```python
from build123d import *

# Parameters (mm, degrees)
F0_R     = 18.527319
F1_DEPTH = 25.4
F3_DEPTH = 77.216
F5_W     = 28.118574
F5_H     = 19.64978
F6_DEPTH = 25.4


with BuildPart() as f1:
    # F0 (on Top) → F1 (new body)
    with BuildSketch(Plane.XY):
        Circle(F0_R)
    extrude(amount=F1_DEPTH)

    # F2 (on face) → F3 (join)
    with BuildSketch(Plane.XY.offset(25.4)):
        Polygon((6.063722, 17.506937), (-9.906806, 15.656205), (-18.417307, 2.016032), (-13.0592, -13.142255), (2.132751, -18.404156), (15.718697, -9.807352), (17.468143, 6.174588), align=None)
    extrude(amount=F3_DEPTH)

    # F5 (on face) → F6 (join)
    with BuildSketch(Plane.XY.offset(102.616)):
        Rectangle(F5_W, F5_H)
    extrude(amount=F6_DEPTH)


solid = f1.part
```
Geometry check sheet. Reference: the model listing, model coordinates, mm. A direction names the side the tool comes from. Coordinates: 2 decimals unless noted, no trailing zeros. Order: outer loops, then holes, each group sorted by start corner. A loop starts at its lowest first (then second) coordinate and runs counter-clockwise, first axis right, second up.
Q1. Thickness scan on probe 1 along Z at (x, y) = (-1, -17); probe 2 along Y at (x, z) = (6, 119.5); probe 3 along X at (y, z) = (-4, 115). Record the ranges inside material, lowest first.
Reply:
probe 1: z = 0 to 102.62
probe 2: y = -9.82 to 9.82
probe 3: x = -14.06 to 14.06
Q2. Tool access check on faces 1 (the face through (-2, 17, 25.4)), 2 (the face through (0, 13, 102.616)), 3 (the face through (-16, -6, 25.4)), 4 (the face through (14.059, 0, 115)), 5 (the face through (8.831, -14.166, 63.467)). Record the directions out of +Z, -Z, +X, -X, +Y, -Y that give a thin tool (end or side, any length) a straight path to the whole face; none if there is none.
Reply:
face 1: +Z, -X, +Y
face 2: +Z, +X, -X, +Y
face 3: +Z, -X, -Y
face 4: +Z, +X, +Y, -Y
face 5: +Z, +X, -Y
Q3. Depth check by flat-ended pin: pin 1 Ø4 at (x, z) = (-4, 38) entering from +Y; pin 2 Ø12 at (x, z) = (12.5, 86) entering from -Y; pin 3 Ø1.4 at (x, y) = (-0.5, 17.5) entering from +Z. Enter the tip coordinate at first touch or a pass-through.
Reply:
pin 1: stops at y = 16.57
pin 2: stops at y = -15.64
pin 3: stops at z = 25.4
Q4. Sectioned sample at B-B on z = 75. Record the cut outline in (x, y), and give its area (3 significant figures).
Reply:
outline: (-18.42, 2.02) - (-13.06, -13.14) - (2.13, -18.4) - (15.72, -9.81) - (17.47, 6.17) - (6.06, 17.51) - (-9.91, 15.66) - close
area: 939 mm2
Q5. Sectioned sample at A-A on x = 0. Record the cut outline in (y, z), and give its area (3 significant figures).
Reply:
outline: (-18.53, 0) - (18.53, 0) - (18.53, 25.4) - (16.8, 25.4) - (16.8, 102.62) - (9.82, 102.62) - (9.82, 128.02) - (-9.82, 128.02) - (-9.82, 102.62) - (-17.67, 102.62) - (-17.67, 25.4) - (-18.53, 25.4) - close
area: 4,100 mm2
Q6. Sectioned sample at D-D on z = 110. Record the cut outline in (x, y), and give its area (3 significant figures).
Reply:
outline: (-14.06, -9.82) - (14.06, -9.82) - (14.06, 9.82) - (-14.06, 9.82) - close
area: 553 mm2
Q7. Sectioned sample at C-C on y = 0. Record the cut outline in (x, z), and give its area (3 significant figures).
Reply:
outline: (-18.53, 0) - (18.53, 0) - (18.53, 25.4) - (16.79, 25.4) - (16.79, 102.62) - (14.06, 102.62) - (14.06, 128.02) - (-14.06, 128.02) - (-14.06, 102.62) - (-17.7, 102.62) - (-17.7, 25.4) - (-18.53, 25.4) - close
area: 4,320 mm2
